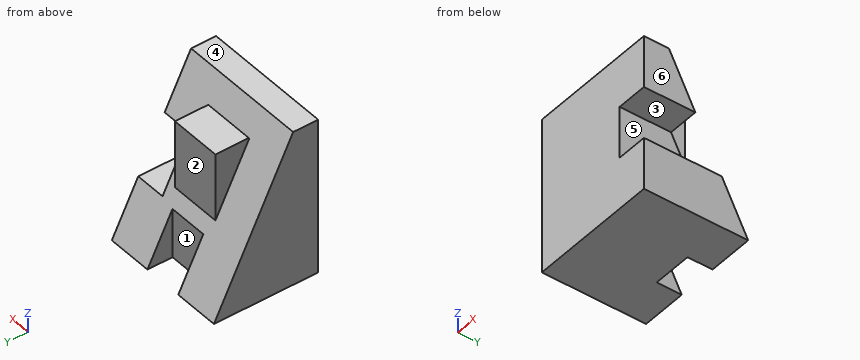
```python
from build123d import *

# Parameters (mm, degrees)
BOSS_EXTRUDE1_DEPTH = 63
CUT_EXTRUDE1_DEPTH  = 15
CUT_EXTRUDE2_REACH  = 111.973
SKETCH3_W           = 19
SKETCH3_H           = 12
BOSS_EXTRUDE2_REACH = 123.973
BOSS_EXTRUDE2_START = -12
SKETCH4_W           = 25
SKETCH4_H           = 16


with BuildPart() as part:
    # Sketch1 → Boss-Extrude1 (new body)
    with BuildSketch(Plane(origin=(0, 0, 0), x_dir=(0, 0, -1), z_dir=(1, 0, 0))):
        Polygon((0, 0), (75, 0), (75, 50), (0, 12), align=None)
    extrude(amount=-BOSS_EXTRUDE1_DEPTH)

    # Sketch2 → Cut-Extrude1 (cut)
    with BuildSketch(Plane(origin=(0, 0, 0), x_dir=(0, 0, -1), z_dir=(1, 0, 0))):
        Polygon((25, 24.666666667), (25, 0), (50, 0), (50, 37.333333333), align=None)
    extrude(amount=-CUT_EXTRUDE1_DEPTH, mode=Mode.SUBTRACT)

    # Sketch3 → Cut-Extrude2 (cut, up to next)
    with BuildSketch(Plane(origin=(0, 0, -75), x_dir=(-1, 0, 0), z_dir=(0, 0, -1)), mode=Mode.PRIVATE) as cut_extrude2_sk1:
        with Locations((31.5, 44)):
            Rectangle(SKETCH3_W, SKETCH3_H)
    cut_extrude2_tool1 = extrude(cut_extrude2_sk1.sketch, amount=-CUT_EXTRUDE2_REACH, mode=Mode.PRIVATE) & part.part
    add(cut_extrude2_tool1.solids().sort_by_distance((-31.5, 44, -75))[0], mode=Mode.SUBTRACT)

    # Boss-Extrude2: up to this plane
    boss_extrude2_end = Plane(origin=(-63, 50, -75), z_dir=(0, 0.8920357760302685, 0.4519647931886695))
    # Sketch4 → Boss-Extrude2 (add, up to the surface)
    with BuildSketch(Plane.XY.offset(BOSS_EXTRUDE2_START), mode=Mode.PRIVATE) as boss_extrude2_sk1:
        with Locations((-31.5, 26.510404023)):
            Rectangle(SKETCH4_W, SKETCH4_H)
    boss_extrude2_tool1 = split(extrude(boss_extrude2_sk1.sketch, amount=-BOSS_EXTRUDE2_REACH, mode=Mode.PRIVATE), bisect_by=boss_extrude2_end, keep=Keep.BOTH, mode=Mode.PRIVATE)
    add(boss_extrude2_tool1.solids().sort_by_distance((-31.5, 26.510404, -12))[0])


solid = part.part
```
Source: CAD feature listing. Evaluate the final solid. Frame: model axes, mm. Face numbers are marked on the shaded views. A direction names the side the tool comes from. Give positions to 0.01 mm unless a question says otherwise; leave off trailing zeros. Loops run counter-clockwise (first coordinate to the right, second up) from the corner with the lowest first, then second, coordinate; pieces in that order, holes last. Notation, with made-up numbers: (5, -13) -> (26, -13) arc R5 cw to (26, -7) -> close; hole circle Ø2 at (-38.75, -38.5). An arc over 180 degrees is marked (long way). Put each result on its own line as item: value. Start each with the question number.
1) Cut plane B-B (z = -69). Return loops of the section in (x, y), then the cut area to 3 significant figures.
2) Material intervals for probe 1 along Z at (x, y) = (-12.5, 10); probe 2 along X at (y, z) = (43, -62); probe 3 along X at (y, z) = (26, -26), sorted ascending.
3) Contact query for flat-ended pins moving along their axis: P1, Ø5, axis at x = -44, z = -53, coming from the +Y side; P2, Ø1, axis at y = 29.5, z = -29, coming from the +X side; P3, Ø8, axis at x = -28.5, y = 23.5, coming from the +Z side. Output: stop coordinate, or through.
4) Draft query along Z for the marked faces 4, 5 and 6. Return one class per face: released by +Z, released by -Z, zero draft, split by the parting line, or undercut.
5) Cut plane A-A (x = -13). Return loops of the section in (y, z), then the cut area to 3 significant figures.
6) Cut plane C-C (y = 6). Return loops of the section in (x, z), then the cut area to 3 significant figures.
7) Cut plane D-D (y = 44.5). Return loops of the section in (x, z).
8) Reachability of the marked faces 1, 2 and 3 from +Z, -Z, +X, -X, +Y, -Y: full face, straight path, thin tool, end or side. Return the list, or none.
Results are:
1. outline: (-63, 0) -> (0, 0) -> (0, 46.96) -> (-22, 46.96) -> (-22, 38) -> (-41, 38) -> (-41, 46.96) -> (-63, 46.96) -> close
1. area: 2,790 mm2
2. probe 1: z = -75 to -50, -25 to 0
2. probe 2: x = -63 to -41, -22 to 0
2. probe 3: x = -44 to -19
3. P1: stops at y = 40.12
3. P2: stops at x = -19
3. P3: stops at z = -12
4. face 4: released by +Z
4. face 5: undercut
4. face 6: zero draft
5. outline: (0, -75) -> (50, -75) -> (37.33, -50) -> (0, -50) -> close; (0, -25) -> (24.67, -25) -> (12, 0) -> (0, 0) -> close
5. area: 1,550 mm2
6. outline: (-63, -75) -> (0, -75) -> (0, -50) -> (-15, -50) -> (-15, -25) -> (0, -25) -> (0, 0) -> (-63, 0) -> close
6. area: 4,350 mm2
7. outline: (-63, -75) -> (-41, -75) -> (-41, -64.14) -> (-63, -64.14) -> close; (-22, -75) -> (0, -75) -> (0, -64.14) -> (-22, -64.14) -> close
8. face 1: +Z, -Z, +Y
8. face 2: +Z, +X, -X, +Y
8. face 3: +X, +Y, -Y
